```python
from build123d import *

# Parameters (mm, degrees)
SKETCH1_W      = 64.008
SKETCH1_H      = 88.9
EXTRUDE1_DEPTH = 6.35
SKETCH2_R      = 2.54
EXTRUDE2_DEPTH = 56.139650126
SKETCH3_R      = 9.525
EXTRUDE4_DEPTH = 56.139650126
SKETCH4_R      = 3.175
EXTRUDE5_DEPTH = 56.139650126


with BuildPart() as part:
    # Sketch1 → Extrude1 (new body)
    with BuildSketch(Plane.XY):
        Rectangle(SKETCH1_W, SKETCH1_H)
    extrude(amount=EXTRUDE1_DEPTH)

    # Sketch2 → Extrude2 (cut, through all)
    with BuildSketch(Plane.XY.offset(6.35)):
        with Locations((-25.4, -19.05)):
            Circle(SKETCH2_R)
        with Locations(Location((25.4, -19.05, 0), (0, 0, 180))):
            Circle(SKETCH2_R)
    extrude(amount=-EXTRUDE2_DEPTH, mode=Mode.SUBTRACT)

    # Sketch3 → Extrude4 (cut, through all)
    with BuildSketch(Plane.XY.offset(6.35)):
        with Locations((0, -19.05)):
            Circle(SKETCH3_R)
    extrude(amount=-EXTRUDE4_DEPTH, mode=Mode.SUBTRACT)

    # Sketch4 → Extrude5 (cut, through all)
    with BuildSketch(Plane.XY.offset(6.35)):
        with Locations((-16.51, 34.29)):
            Circle(SKETCH4_R)
        with Locations(Location((16.51, 34.29, 0), (0, 0, 180))):
            Circle(SKETCH4_R)
    extrude(amount=-EXTRUDE5_DEPTH, mode=Mode.SUBTRACT)


solid = part.part
```
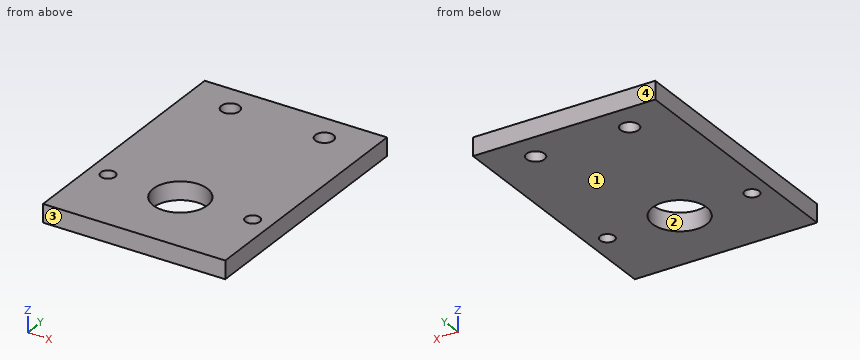
CAD build for the part. Positions are in the model's coordinates, mm. Face numbers are marked on the shaded views. Give positions to 0.01 mm unless a question says otherwise; leave off trailing zeros. Write each loop counter-clockwise with the first axis right and the second up, starting at its lowest first coordinate (ties: lowest second). Pieces come first, ordered by that corner, then holes. Notation, with made-up numbers: (-13, -17) -> (5, -17) arc R29 cw to (5, 8) -> close; hole circle Ø5 at (65.5, -37). An arc over 180 degrees is marked (long way). Write each question's results on one line, items separated by ' | '.
1. Cut at B-B, the plane y = 34.29. Write the cut outline in (x, z) (3 decimals).
Geometry check:
outline: (-32.004, 0) -> (-19.685, 0) -> (-19.685, 6.35) -> (-32.004, 6.35) -> close; (-13.335, 0) -> (13.335, 0) -> (13.335, 6.35) -> (-13.335, 6.35) -> close; (19.685, 0) -> (32.004, 0) -> (32.004, 6.35) -> (19.685, 6.35) -> close
2. Cut at C-C, the plane z = 4.25. Write the cut outline in (x, y) (3 decimals).
Geometry check:
outline: (-32.004, -44.45) -> (32.004, -44.45) -> (32.004, 44.45) -> (-32.004, 44.45) -> close; hole circle Ø5.08 at (-25.4, -19.05); hole circle Ø6.35 at (-16.51, 34.29); hole circle Ø19.05 at (0, -19.05); hole circle Ø6.35 at (16.51, 34.29); hole circle Ø5.08 at (25.4, -19.05)
3. Wall check: probe 1 along Y at (x, z) = (16.51, 2.5) (3 decimals); probe 2 along Y at (x, z) = (-25.4, 4.5); probe 3 along X at (y, z) = (-15, 5). Give the ranges that are in metal, low to high. Write a range as [from, to].
Geometry check:
probe 1: [-44.45, 31.115], [37.465, 44.45] | probe 2: [-44.45, -21.59], [-16.51, 44.45] | probe 3: [-32, -8.62], [8.62, 32]
4. Two-plate mould, pull along Y, no slides. Class the marked faces 1, 2, 3 and 4: pulls with the +Y half, pulls with the -Y half, needs draft (parallel to the pull), parting line crosses it, or undercut.
Geometry check:
face 1: needs draft | face 2: undercut | face 3: pulls with the -Y half | face 4: pulls with the +Y half
5. Cut at A-A, the plane x = 16.51. Write the cut outline in (y, z) (3 decimals), then the cut area to 3 significant figures.
Geometry check:
outline: (-44.45, 0) -> (31.115, 0) -> (31.115, 6.35) -> (-44.45, 6.35) -> close; (37.465, 0) -> (44.45, 0) -> (44.45, 6.35) -> (37.465, 6.35) -> close | area: 524 mm²
6. Cut at D-D, the plane y = -14. Write the cut outline in (x, z).
Geometry check:
outline: (-32, 0) -> (-8.08, 0) -> (-8.08, 6.35) -> (-32, 6.35) -> close; (8.08, 0) -> (32, 0) -> (32, 6.35) -> (8.08, 6.35) -> close
